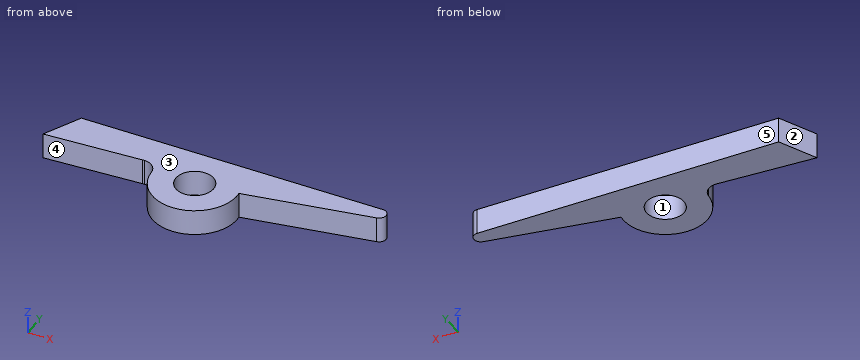
```python
from build123d import *

# Parameters (mm, degrees)
SKETCH1_R           = 4
BOSS_EXTRUDE1_DEPTH = 5.5


with BuildPart() as part:
    # Sketch1 → Boss-Extrude1 (new body)
    with BuildSketch(Plane.XY):
        with BuildLine():
            ThreePointArc((-12.335531392, 2.238518271), (-12.156668127, 2.254624752), (-11.9771616, 2.26))
            ThreePointArc((-11.9771616, 2.26), (-9.922289344, 1.445749302), (-8.982871201, -0.554999992))
            ThreePointArc((-8.982871201, -0.554999992), (0.778132217, -8.966298582), (8.944184276, 1.000783512))
            Line((8.944184276, 1.000783512), (35.778917143, 6.025625378))
            ThreePointArc((35.778917143, 6.025625378), (36.996418316, 7.638632727), (35.5028384, 9))
            Line((35.5028384, 9), (-28.9971616, 9))
            Line((-28.9971616, 9), (-32.9971616, 1))
            Line((-32.9971616, 1), (-12.335531392, 2.238518271))
        make_face()
        Circle(SKETCH1_R, mode=Mode.SUBTRACT)
    extrude(amount=BOSS_EXTRUDE1_DEPTH)


solid = part.part
```
Model file for the job. Use its own axes, mm. Face numbers are marked on the shaded views. A direction names the side the tool comes from. Round coordinates to 2 decimals unless told otherwise and drop trailing zeros. Order: outer loops, then holes, each group sorted by start corner. A loop starts at its lowest first (then second) coordinate and runs counter-clockwise, first axis right, second up. Notation, with made-up numbers: M 10.25,47 L 37.25,47 A31 ccw 37.25,84 Z; hole C -8.5,31 d9. An arc over 180 degrees is marked long. Use CSV: the item, a comma, the result in double quotes.
Item 1: Saw through at A-A (x = 0). List the corners of the cut face in (y, z), plus the area to 3 significant figures.
Worked answers:
outline,"M -9,0 L -4,0 L -4,5.5 L -9,5.5 Z; M 4,0 L 9,0 L 9,5.5 L 4,5.5 Z"
area,"55.0 mm²"
Item 2: Pull direction Y, two halves, no side cores. Call the marked faces 1, 2 and 3: released by +Y, released by -Y, zero draft, split by the parting line, or undercut.
Worked answers:
face 1,"undercut"
face 2,"released by +Y"
face 3,"zero draft"
Item 3: Saw through at C-C (y = -2.75). List the corners of the cut face in (x, z).
Worked answers:
outline,"M -8.57,0 L -2.9,0 L -2.9,5.5 L -8.57,5.5 Z; M 2.9,0 L 8.57,0 L 8.57,5.5 L 2.9,5.5 Z"
Item 4: Pin check, flat tips, straight feed: pin 1 (2 mm diameter, centred on y = -0.5, z = 0.5, fed in from -X); pin 2 (1 mm diameter, centred on y = -4.5, z = 4.5, fed in from -X). Stop position of each tip, or through.
Worked answers:
pin 1,"x = -9.25"
pin 2,"x = -8.06"
Item 5: Which spindle directions (+Z, -Z, +X, -X, +Y, -Y) get a long thin tool onto all of the face, cutting with end or side? Do the marked faces 4 and 5. Say none if no direction does.
Worked answers:
face 4,"+Z, -Z, -Y"
face 5,"+Z, -Z, +X, -X, +Y"
Item 6: Saw through at D-D (x = -16). List the corners of the cut face in (y, z).
Worked answers:
outline,"M 2.02,0 L 9,0 L 9,5.5 L 2.02,5.5 Z"
Item 7: Probe probe 1 along Y at (x, z) = (0, 3.1); probe 2 along X at (y, z) = (0.75, 1.05); probe 3 along X at (y, z) = (-2, 1.4). List the from-to ranges inside material, lowest first.
Worked answers:
probe 1,"-9 to -4, 4 to 9"
probe 2,"-9.37 to -3.93, 3.93 to 8.97"
probe 3,"-8.77 to -3.46, 3.46 to 8.77"
Item 8: Saw through at B-B (z = 2.6). List the corners of the cut face in (x, y) (3 decimals), plus the area to 3 significant figures.
Worked answers:
outline,"M -32.997,1 L -12.336,2.239 A3 cw -8.983,-0.555 A9 ccw long 8.944,1.001 L 35.779,6.026 A1.5 ccw 35.503,9 L -28.997,9 Z; hole C 0,0 d8"
area,"549 mm²"
